```python
from build123d import *

# Parameters (mm, degrees)
SKETCH1_R           = 4
SKETCH1_R_2         = 2.5
BOSS_EXTRUDE1_DEPTH = 7
SKETCH2_R           = 4
SKETCH2_R_2         = 2.5
BOSS_EXTRUDE2_DEPTH = 7
BOSS_EXTRUDE3_DEPTH = 14


with BuildPart() as part:
    # Sketch1 → Boss-Extrude1 (new body)
    with BuildSketch(Plane(origin=(0, 0, 0), x_dir=(1, 0, 0), z_dir=(0, 1, 0))):
        with Locations(Location((0.5, 0, 0), (0, 0, 270))):
            Circle(SKETCH1_R)
        with Locations(Location((0, 0, 0), (0, 0, 270))):
            Circle(SKETCH1_R_2, mode=Mode.SUBTRACT)
    extrude(amount=BOSS_EXTRUDE1_DEPTH)

    # Sketch2 → Boss-Extrude2 (add)
    with BuildSketch(Plane(origin=(0, 7, 0), x_dir=(1, 0, 0), z_dir=(0, 1, 0))):
        with Locations(Location((-0.5, 0, 0), (0, 0, 82.819244219))):
            Circle(SKETCH2_R)
        with Locations(Location((0, 0, 0), (0, 0, 270))):
            Circle(SKETCH2_R_2, mode=Mode.SUBTRACT)
    extrude(amount=BOSS_EXTRUDE2_DEPTH)

    # Sketch3 → Boss-Extrude3 (add, through all)
    with BuildSketch(Plane(origin=(0, 14, 0), x_dir=(1, 0, 0), z_dir=(0, 1, 0))):
        with BuildLine():
            Line((1.5, 2), (1.5, -2))
            ThreePointArc((1.5, -2), (2.5, 0), (1.5, 2))
        make_face()
    extrude(amount=-BOSS_EXTRUDE3_DEPTH)


solid = part.part
```
CAD build for the part. Positions are in the model's coordinates, mm. A direction names the side the tool comes from. Round coordinates to 2 decimals unless told otherwise and drop trailing zeros. Order: outer loops, then holes, each group sorted by start corner. A loop starts at its lowest first (then second) coordinate and runs counter-clockwise, first axis right, second up. Notation, with made-up numbers: (58.5, 36) - (70.5, 36) arc R19 cw to (70.5, 43) - close; hole circle Ø11 at (5.5, -13). An arc over 180 degrees is marked (long way). Answer as CSV lines item,"result". Start each with the question number.
1. Saw through at C-C, the plane y = 5.75. Write the cut outline in (x, z), and give its area (3 significant figures).
2. Saw through at B-B, the plane x = -2.25. Write the cut outline in (y, z).
3. Saw through at D-D, the plane z = -3.25. Write the cut outline in (x, y), and give its area (3 significant figures).
4. Saw through at A-A, the plane z = 0. Write the cut outline in (x, y).
5. Drill centre lines: L1, parallel to Z at x = -0.75, y = 3; L2, parallel to Z at x = 0, y = 3; L3, parallel to Y at x = 3.5, z = -1.5. Where is each one in solid material? Low to high. Write a range as [from, to].
6. Pin check, flat tips, straight feed: pin 1 (1.5 mm diameter, centred on x = -2.5, y = 3.5, fed in from +Z); pin 2 (3 mm diameter, centred on y = 7, z = -3, fed in from -X); pin 3 (4 mm diameter, centred on y = 12, z = 2.5, fed in from -X). Stop position of each tip, or through.
7. Pull direction Z, two halves, no side cores. Call faces 1 (the face through (-3.405, 3.451, -0.867)), 2 (the face through (-2.5, 6.9, -0.1)), 3 (the face through (2, 0, 0)): +Z half, -Z half, draft (parallel to the pull), parting line (faces both ways), or undercut.
8. Tool access for faces 4 (the face through (1.5, 7, 0)), 5 (the face through (4, 7, 0)), 6 (the face through (3.266, 10.451, 1.348)): list every direction of +Z, -Z, +X, -X, +Y, -Y with a clear straight run to the whole face (end or side of a thin tool).
Model answer:
1,outline,"circle Ø8 at (0.5, 0); hole (1.5, -2) - (1.5, 2) arc R2.5 ccw (long way) to start"
1,area,"33.4 mm²"
2,outline,"(0, -2.9) - (7, -2.9) - (7, -3.6) - (14, -3.6) - (14, -1.09) - (0, -1.09) - close; (0, 1.09) - (14, 1.09) - (14, 3.6) - (7, 3.6) - (7, 2.9) - (0, 2.9) - close"
3,outline,"(-2.83, 7) - (-1.83, 7) - (-1.83, 0) - (2.83, 0) - (2.83, 7) - (1.83, 7) - (1.83, 14) - (-2.83, 14) - close"
3,area,"65.3 mm²"
4,outline,"(-4.5, 7) - (-3.5, 7) - (-3.5, 0) - (-2.5, 0) - (-2.5, 14) - (-4.5, 14) - close; (1.5, 0) - (4.5, 0) - (4.5, 7) - (3.5, 7) - (3.5, 14) - (1.5, 14) - close"
5,L1,"z = [-3.8, -2.38], [2.38, 3.8]"
5,L2,"z = [-3.97, -2.5], [2.5, 3.97]"
5,L3,"y = [0, 7]"
6,pin 1,"stops at z = 3.31"
6,pin 2,"stops at x = -4.21"
6,pin 3,"stops at x = -4.47"
7,face 1,"parting line"
7,face 2,"undercut"
7,face 3,"draft"
8,face 4,"+Y, -Y"
8,face 5,"+X, +Y"
8,face 6,"+Y"
